```python
from build123d import *

# Parameters (mm, degrees)
F0_W     = 51.809754
F0_H     = 79.682095
F0_W_2   = 41.31664
F0_H_2   = 67.549428
F0_W_3   = 62.63078
F0_W_4   = 52.465571
F0_H_3   = 66.565698
F1_DEPTH = 12.7
F2_W     = 137.722135
F2_H     = 92.470575
F3_DEPTH = 2.54
F4_W     = 12.132665
F4_H     = 65.58197
F5_DEPTH = 83.312
F6_R     = 5.504968
F7_DEPTH = 108.712


with BuildPart() as f1:
    # F0 (on Front) → F1 (new body)
    with BuildSketch(Plane.XZ):
        with Locations((-25.904877, 12.460576)):
            Rectangle(F0_W, F0_H)
        with Locations((-26.560696, 12.624529)):
            Rectangle(F0_W_2, F0_H_2, mode=Mode.SUBTRACT)
        with Locations((31.31539, 12.460576)):
            Rectangle(F0_W_3, F0_H)
        with Locations((31.479344, 12.132664)):
            Rectangle(F0_W_4, F0_H_3, mode=Mode.SUBTRACT)
    extrude(amount=F1_DEPTH)

    # F2 (on Front) → F3 (join)
    with BuildSketch(Plane.XZ):
        with Locations((6.230287, 12.296619)):
            Rectangle(F2_W, F2_H)
    extrude(amount=F3_DEPTH)

    # F4 (on Front) → F5 (join)
    with BuildSketch(Plane.XZ):
        with Locations((-0.163952, 12.296621)):
            Rectangle(F4_W, F4_H)
    extrude(amount=F5_DEPTH)

    # F6 (on Front) → F7 (join)
    with BuildSketch(Plane.XZ):
        with Locations((0, 19.058177)):
            Circle(F6_R)
    extrude(amount=F7_DEPTH)


solid = f1.part
```
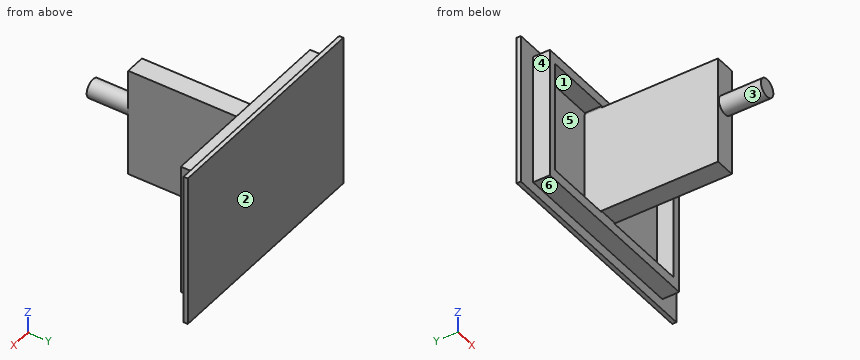
Check sheet for the modelled part. Datum: model origin and axes. Units: mm. Face numbers are marked on the shaded views. A direction names the side the tool comes from. Round coordinates to 2 decimals unless told otherwise and drop trailing zeros. Order: outer loops, then holes, each group sorted by start corner. A loop starts at its lowest first (then second) coordinate and runs counter-clockwise, first axis right, second up.
1) Tool access check on the marked faces 1 and 2. Record the directions out of +Z, -Z, +X, -X, +Y, -Y that give a thin tool (end or side, any length) a straight path to the whole face; none if there is none.
2) Mould release check, pull along X, two halves, no side actions. Record for the marked faces 3, 4, 5 and 6: +X half, -X half, draft (parallel to the pull), parting line (faces both ways), or undercut.
3) Section check B-B (z = 26.5). Record the boundary of the cut face in (x, y), and give its area (3 significant figures).
4) Section check C-C (x = -44.5). Record the boundary of the cut face in (y, z), and give its area (3 significant figures).
5) Section check A-A (x = 0). Record the boundary of the cut face in (y, z).
6) Go/stop test with flat-tipped pins: pin 1 Ø8 at (y, z) = (-8, 27) entering from +X; pin 2 Ø3 at (x, y) = (16, -8.5) entering from -Z; pin 3 Ø5 at (y, z) = (-64.5, -10.5) entering from -X. Record where each tip stops, or that it passes through.
7) Scan lines: line 1 (Z direction, x = -23.5, y = -12); line 2 (Y direction, x = -22, z = 38); line 3 (X direction, y = -70.5, z = 13.5). Record each from-to range of solid material in increasing order.
Result:
1. face 1: -Y
1. face 2: +Z, -Z, +X, -X, +Y
2. face 3: parting line
2. face 4: -X half
2. face 5: undercut
2. face 6: draft
3. outline: (-62.63, -2.54) - (-51.81, -2.54) - (-51.81, -12.7) - (-47.22, -12.7) - (-47.22, -2.54) - (-6.23, -2.54) - (-6.23, -83.31) - (5.9, -83.31) - (5.9, -2.54) - (57.71, -2.54) - (57.71, -12.7) - (62.63, -12.7) - (62.63, -2.54) - (75.09, -2.54) - (75.09, 0) - (-62.63, 0) - close
3. area: 1,430 mm2
4. outline: (-12.7, -27.38) - (-2.54, -27.38) - (-2.54, -33.94) - (0, -33.94) - (0, 58.53) - (-2.54, 58.53) - (-2.54, 52.3) - (-12.7, 52.3) - (-12.7, 46.4) - (-2.54, 46.4) - (-2.54, -21.15) - (-12.7, -21.15) - close
4. area: 358 mm2
5. outline: (-108.71, 13.55) - (-83.31, 13.55) - (-83.31, -20.49) - (-12.7, -20.49) - (-12.7, -27.38) - (-2.54, -27.38) - (-2.54, -33.94) - (0, -33.94) - (0, 58.53) - (-2.54, 58.53) - (-2.54, 52.3) - (-12.7, 52.3) - (-12.7, 45.09) - (-83.31, 45.09) - (-83.31, 24.56) - (-108.71, 24.56) - close
6. pin 1: stops at x = 62.63
6. pin 2: stops at z = -27.38
6. pin 3: stops at x = -6.23
7. line 1: z = -27.38 to -21.15, 46.4 to 52.3
7. line 2: y = -2.54 to 0
7. line 3: x = -6.23 to 5.9
